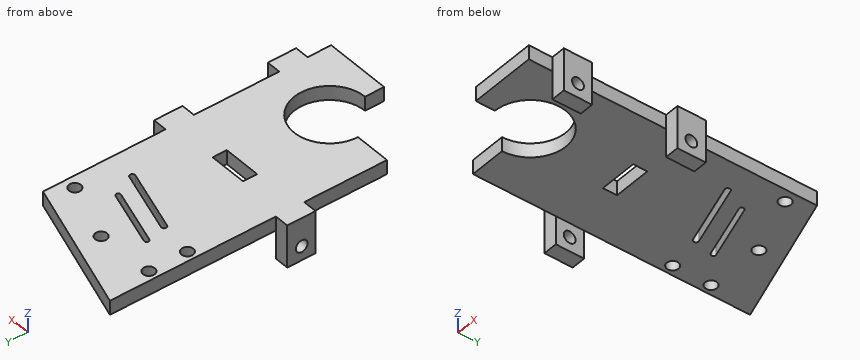
```python
from build123d import *

# Parameters (mm, degrees)
SKETCH1_W                 = 29.13
SKETCH1_H                 = 2
BOSS_EXTRUDE1_DEPTH       = 45.22
SKETCH15_W                = 3.835
SKETCH15_H                = 2
BOSS_EXTRUDE7_DEPTH       = 25.02
CUT_EXTRUDE5_DEPTH        = 4
SKETCH19_W                = 2
SKETCH19_H                = 6
BOSS_EXTRUDE9_DEPTH       = 3
SKETCH20_W                = 3
SKETCH20_H                = 6
BOSS_EXTRUDE10_DEPTH      = 6
SKETCH21_R                = 1.25
CUT_EXTRUDE6_DEPTH        = 6
CUT_EXTRUDE10_DEPTH       = 4
SKETCH27_R                = 1.25
CUT_EXTRUDE13_DEPTH       = 5
CUT_EXTRUDE16_DEPTH       = 4.86
CUT_EXTRUDE17_DEPTH       = 4
CUT_EXTRUDE20_DEPTH       = 15
SKETCH28_R                = 1.25
CUT_EXTRUDE23_DEPTH       = 5
SKETCH32_R                = 1.25
CUT_EXTRUDE25_DEPTH       = 5
SKETCH38_W                = 2
SKETCH38_H                = 6
BOSS_EXTRUDE11_DEPTH      = 3
SKETCH39_W                = 3
SKETCH39_H                = 6
BOSS_EXTRUDE12_DEPTH      = 6
SKETCH40_R                = 1.250000005
CUT_EXTRUDE26_DEPTH       = 6
SKETCH51_W                = 2
SKETCH51_H                = 6
BOSS_EXTRUDE15_DEPTH      = 3
SKETCH52_W                = 3
SKETCH52_H                = 6
BOSS_EXTRUDE16_DEPTH      = 6
SKETCH53_R                = 1.249999995
CUT_EXTRUDE28_DEPTH       = 6
BOSS_EXTRUDE17_DEPTH      = 1
BOSS_EXTRUDE17_DEPTH_BACK = 2
CUT_EXTRUDE29_DEPTH       = 1
CUT_EXTRUDE29_DEPTH_BACK  = 2
SKETCH54_3_R              = 7.5
BOSS_EXTRUDE18_DEPTH      = 1
BOSS_EXTRUDE18_DEPTH_BACK = 2
SKETCH55_R                = 1.25
CUT_EXTRUDE30_DEPTH       = 10


with BuildPart() as part:
    # Sketch1 → Boss-Extrude1 (new body)
    with BuildSketch(Plane(origin=(0, 0, 0), x_dir=(1, 0, 0), z_dir=(0, 1, 0))):
        with Locations((-35.580481579, -22.688974349)):
            Rectangle(SKETCH1_W, SKETCH1_H)
    extrude(amount=BOSS_EXTRUDE1_DEPTH)

    # Sketch15 → Boss-Extrude7 (add)
    with BuildSketch(Plane.XZ):
        with Locations((-22.932981579, 22.688974349)):
            Rectangle(SKETCH15_W, SKETCH15_H)
    extrude(amount=BOSS_EXTRUDE7_DEPTH)

    # Sketch16 → Cut-Extrude5 (cut)
    with BuildSketch(Plane.XY.offset(23.688974349)):
        Polygon((-24.850481579, 0), (-21.015481579, -25.02), (-24.850481579, -25.02), align=None)
    extrude(amount=-CUT_EXTRUDE5_DEPTH, mode=Mode.SUBTRACT)

    # Sketch19 → Boss-Extrude9 (add)
    with BuildSketch(Plane(origin=(-21.015481579, 0, 0), x_dir=(0, 0, -1), z_dir=(1, 0, 0))):
        with Locations((-22.688974349, -17.02)):
            Rectangle(SKETCH19_W, SKETCH19_H)
    extrude(amount=BOSS_EXTRUDE9_DEPTH)

    # Sketch20 → Boss-Extrude10 (add)
    with BuildSketch(Plane(origin=(0, 0, 21.688974349), x_dir=(-1, 0, 0), z_dir=(0, 0, -1))):
        with Locations((19.515481579, -17.02)):
            Rectangle(SKETCH20_W, SKETCH20_H)
    extrude(amount=BOSS_EXTRUDE10_DEPTH)

    # Sketch21 → Cut-Extrude6 (cut)
    with BuildSketch(Plane(origin=(-18.015481579, 0, 0), x_dir=(0, 0, -1), z_dir=(1, 0, 0))):
        with Locations((-18.688974344, -17.012020694)):
            Circle(SKETCH21_R)
    extrude(amount=-CUT_EXTRUDE6_DEPTH, mode=Mode.SUBTRACT)

    # Sketch24 → Cut-Extrude10 (cut)
    with BuildSketch(Plane.XY.offset(23.688974349)):
        Polygon((-21.015481579, 45.22), (-21.015481579, 37.57), (-50.145481579, 45.22), align=None)
    extrude(amount=-CUT_EXTRUDE10_DEPTH, mode=Mode.SUBTRACT)

    # Sketch27 → Cut-Extrude13 (cut)
    with BuildSketch(Plane.XY.offset(23.688974349)):
        with Locations((-48.155481578, 35.325814088)):
            Circle(SKETCH27_R)
        with Locations((-48.155481579, 27.181192798)):
            Circle(SKETCH27_R)
    extrude(amount=-CUT_EXTRUDE13_DEPTH, mode=Mode.SUBTRACT)

    # Sketch35 → Cut-Extrude16 (cut)
    with BuildSketch(Plane.XY.offset(23.688974349)):
        Polygon((-21.015481579, 35.99), (-21.015481579, 37.57), (-50.145481579, 45.22), align=None)
    extrude(amount=-CUT_EXTRUDE16_DEPTH, mode=Mode.SUBTRACT)

    # Sketch36 → Cut-Extrude17 (cut)
    with BuildSketch(Plane.XY.offset(23.688974349)):
        Polygon((-50.145481579, 45.22), (-50.145481579, 45.18), (-21.015481579, 35.99), align=None)
    extrude(amount=-CUT_EXTRUDE17_DEPTH, mode=Mode.SUBTRACT)


with BuildPart() as body_2:
    # Mirror1: mirrored copy
    add(part.part.mirror(Plane(origin=(0, 0, 15.688974349), x_dir=(1, 0, 0), z_dir=(0, 0, -1))))

    # Sketch37 → Cut-Extrude20 (cut)
    with BuildSketch(Plane(origin=(0, 0, 7.688974349), x_dir=(-1, 0, 0), z_dir=(0, 0, -1))):
        with BuildLine():
            Line((29.422391304, 27.369440111), (41.452993211, 31.026802565))
            ThreePointArc((41.452993211, 31.026802565), (42.065476612, 30.699897808), (41.738571855, 30.087414406))
            Line((41.738571855, 30.087414406), (29.707969948, 26.430051952))
            ThreePointArc((29.707969948, 26.430051952), (29.095486546, 26.75695671), (29.422391304, 27.369440111))
        make_face()
        with BuildLine():
            Line((26.963881394, 22.478846245), (40.405895564, 26.565285004))
            ThreePointArc((40.405895564, 26.565285004), (41.083801623, 26.203461785), (40.721978404, 25.525555725))
            Line((40.721978404, 25.525555725), (27.279964235, 21.439116966))
            ThreePointArc((27.279964235, 21.439116966), (26.602058175, 21.800940185), (26.963881394, 22.478846245))
        make_face()
    extrude(amount=-CUT_EXTRUDE20_DEPTH, mode=Mode.SUBTRACT)


with BuildPart() as body_2_2:
    # Mirror2: mirrored copy
    add(body_2.part.mirror(Plane.XY.offset(15.688974349)))

    # Sketch28 → Cut-Extrude23 (cut)
    with BuildSketch(Plane.XY.offset(23.688974349)):
        with Locations((-23.525481579, 31.253503442)):
            Circle(SKETCH28_R)
    extrude(amount=-CUT_EXTRUDE23_DEPTH, mode=Mode.SUBTRACT)

    # Sketch32 → Cut-Extrude25 (cut)
    with BuildSketch(Plane.XY.offset(23.688974349)):
        with Locations((-36.114456583, 35.789812976)):
            Circle(SKETCH32_R)
    extrude(amount=-CUT_EXTRUDE25_DEPTH, mode=Mode.SUBTRACT)

    # Sketch38 → Boss-Extrude11 (add)
    with BuildSketch(Plane.ZY.offset(50.145481579)):
        with Locations((22.688974349, 7.042669101)):
            Rectangle(SKETCH38_W, SKETCH38_H)
    extrude(amount=BOSS_EXTRUDE11_DEPTH)

    # Sketch39 → Boss-Extrude12 (add)
    with BuildSketch(Plane(origin=(0, 0, 21.688974349), x_dir=(-1, 0, 0), z_dir=(0, 0, -1))):
        with Locations((51.645481579, 7.042669101)):
            Rectangle(SKETCH39_W, SKETCH39_H)
    extrude(amount=BOSS_EXTRUDE12_DEPTH)

    # Sketch40 → Cut-Extrude26 (cut)
    with BuildSketch(Plane.ZY.offset(53.145481579)):
        with Locations((18.688974344, 6.98)):
            Circle(SKETCH40_R)
    extrude(amount=-CUT_EXTRUDE26_DEPTH, mode=Mode.SUBTRACT)

    # Sketch51 → Boss-Extrude15 (add)
    with BuildSketch(Plane(origin=(-21.015481579, 0, 0), x_dir=(0, 0, -1), z_dir=(1, 0, 0))):
        with Locations((-22.688974349, 7.042669101)):
            Rectangle(SKETCH51_W, SKETCH51_H)
    extrude(amount=BOSS_EXTRUDE15_DEPTH)

    # Sketch52 → Boss-Extrude16 (add)
    with BuildSketch(Plane(origin=(0, 0, 21.688974349), x_dir=(-1, 0, 0), z_dir=(0, 0, -1))):
        with Locations((19.515481579, 7.042669101)):
            Rectangle(SKETCH52_W, SKETCH52_H)
    extrude(amount=BOSS_EXTRUDE16_DEPTH)

    # Sketch53 → Cut-Extrude28 (cut)
    with BuildSketch(Plane(origin=(-18.015481579, 0, 0), x_dir=(0, 0, -1), z_dir=(1, 0, 0))):
        with Locations(Location((-18.688974344, 6.98, 0), (0, 0, 180))):
            Circle(SKETCH53_R)
    extrude(amount=-CUT_EXTRUDE28_DEPTH, mode=Mode.SUBTRACT)

    # Sketch54 → Boss-Extrude17 (add, two sides: drawn at the far end of the back side and taken through both)
    with BuildSketch(Plane.XY.offset(23.688974349).offset(-BOSS_EXTRUDE17_DEPTH_BACK)):
        Polygon((-50.145481579, 0), (-50.145481579, -13.48149478), (-34.98674486, -13.48149478), (-34.98674486, -25.02), (-21.015481579, -25.02), (-24.850481579, 0), align=None)
    extrude(amount=BOSS_EXTRUDE17_DEPTH + BOSS_EXTRUDE17_DEPTH_BACK)

    # Sketch54<3> → Cut-Extrude29 (cut, two sides: drawn at the far end of the back side and taken through both)
    with BuildSketch(Plane.XY.offset(23.688974349).offset(-CUT_EXTRUDE29_DEPTH_BACK)):
        with Locations((-34.98674486, -13.48149478)):
            Circle(SKETCH54_3_R)
    extrude(amount=CUT_EXTRUDE29_DEPTH + CUT_EXTRUDE29_DEPTH_BACK, mode=Mode.SUBTRACT)

    # Sketch55 → Boss-Extrude18 (add, two sides: drawn at the far end of the back side and taken through both)
    with BuildSketch(Plane.XY.offset(23.688974349).offset(-BOSS_EXTRUDE18_DEPTH_BACK)):
        Polygon((-50.145481579, 45.18), (-50.145481579, 10.042669101), (-53.145481579, 10.042669101), (-53.145481579, 4.042669101), (-50.145481579, 4.042669101), (-50.145481579, 0), (-24.850481579, 0), (-21.015481579, -25.02), (-21.015481579, -20.02), (-18.015481579, -20.02), (-18.015481579, -14.02), (-21.015481579, -14.02), (-21.015481579, 4.042669101), (-18.015481579, 4.042669101), (-18.015481579, 10.042669101), (-21.015481579, 10.042669101), (-21.015481579, 35.99), align=None)
        with Locations((-23.525481579, 31.253503442)):
            Circle(SKETCH55_R, mode=Mode.SUBTRACT)
        with Locations((-36.114456583, 35.789812976)):
            Circle(SKETCH55_R, mode=Mode.SUBTRACT)
        with Locations((-48.155481578, 35.325814088)):
            Circle(SKETCH55_R, mode=Mode.SUBTRACT)
        with Locations((-48.155481579, 27.181192798)):
            Circle(SKETCH55_R, mode=Mode.SUBTRACT)
        with BuildLine():
            Line((-41.453555794, 31.024951992), (-29.422953887, 27.367589538))
            ThreePointArc((-29.422953887, 27.367589538), (-29.097337119, 26.757519293), (-29.707407364, 26.431902525))
            Line((-29.707407364, 26.431902525), (-41.738009272, 30.089264979))
            ThreePointArc((-41.738009272, 30.089264979), (-42.063626039, 30.699335224), (-41.453555794, 31.024951992))
        make_face(mode=Mode.SUBTRACT)
        with BuildLine():
            Line((-27.280327459, 21.437922169), (-40.722341628, 25.524360928))
            ThreePointArc((-40.722341628, 25.524360928), (-41.08499642, 26.203825009), (-40.405532339, 26.566479801))
            Line((-40.405532339, 26.566479801), (-26.96351817, 22.480041042))
            ThreePointArc((-26.96351817, 22.480041042), (-26.600863378, 21.800576961), (-27.280327459, 21.437922169))
        make_face(mode=Mode.SUBTRACT)
    extrude(amount=BOSS_EXTRUDE18_DEPTH + BOSS_EXTRUDE18_DEPTH_BACK)

    # Sketch56 → Cut-Extrude30 (cut)
    with BuildSketch(Plane.XY.offset(24.688974349)):
        Polygon((-31.58048158, 8.542669101), (-35.580481579, 8.542669101), (-39.58048158, 8.542669101), (-39.58048158, 5.542669101), (-31.58048158, 5.542669101), align=None)
    extrude(amount=-CUT_EXTRUDE30_DEPTH, mode=Mode.SUBTRACT)


solid = body_2_2.part
```
Read the model definition and answer for the solid it produces. Units are mm, in the model's axes. Coordinates: 2 decimals unless noted, no trailing zeros. Write each loop counter-clockwise with the first axis right and the second up, starting at its lowest first coordinate (ties: lowest second). Pieces come first, ordered by that corner, then holes. Notation, with made-up numbers: (78, 15.5) -> (130, 15.5) arc R17 ccw to (130, 45.5) -> close; hole circle Ø8 at (-35.75, 8). An arc over 180 degrees is marked (long way). Answer as a JSON object with one key per item and string values.
Q1. Consider line 1 (Z direction, x = -40, y = 31); line 2 (X direction, y = 9.5, z = 19.75); line 3 (X direction, y = 1, z = 23.75). Determine where each line is inside the solid, lowest interval first. Write a range as [from, to].
The answers:
{"line 1": "z = [21.69, 24.69]", "line 2": "x = [-53.15, -50.15], [-21.02, -18.02]", "line 3": "x = [-50.15, -21.02]"}
Q2. The part is cut by section A-A on y = 6.98. Give the vertices of the cut face in (x, z), then the cut area to 3 significant figures.
The answers:
{"outline": "(-53.15, 15.69) -> (-50.15, 15.69) -> (-50.15, 17.44) -> (-53.15, 17.44) -> close; (-53.15, 19.94) -> (-50.15, 19.94) -> (-50.15, 21.69) -> (-39.58, 21.69) -> (-39.58, 24.69) -> (-53.15, 24.69) -> close; (-31.58, 21.69) -> (-21.02, 21.69) -> (-21.02, 19.94) -> (-18.02, 19.94) -> (-18.02, 24.69) -> (-31.58, 24.69) -> close; (-21.02, 15.69) -> (-18.02, 15.69) -> (-18.02, 17.44) -> (-21.02, 17.44) -> close", "area": "102 mm2"}
Q3. Flat-ended cylindrical pins translate along their axes: pin 1 Ø0.9 at (x, z) = (-19.5, 21) entering from +Y; pin 2 Ø1.5 at (y, z) = (-23, 23.5) entering from +X; pin 3 Ø5 at (x, z) = (-43.5, 22.5) entering from -Y; pin 4 Ø3.5 at (y, z) = (6.98, 18.69) entering from -X. Find the tip coordinate at first contact, or state that the pin passes through.
The answers:
{"pin 1": "stops at y = 10.04", "pin 2": "stops at x = -21.02", "pin 3": "stops at y = -13.48", "pin 4": "stops at x = -53.15"}
Q4. The part is cut by section C-C on x = -34. Give the number of separate pieces and of enclosed holes in the cut face, then the cut area to 3 significant figures.
The answers:
{"separate pieces": "5", "enclosed holes": "0", "area": "135 mm2"}
Q5. The part is cut by section B-B on x = -19.5. Give the vertices of the cut face in (y, z).
The answers:
{"outline": "(-20.02, 15.69) -> (-14.02, 15.69) -> (-14.02, 24.69) -> (-20.02, 24.69) -> close; (4.04, 15.69) -> (10.04, 15.69) -> (10.04, 24.69) -> (4.04, 24.69) -> close; hole circle Ø2.5 at (-17.01, 18.69); hole circle Ø2.5 at (6.98, 18.69)"}
